from build123d import *

# Parameters (mm, degrees)
F1_DEPTH = 25.4
F3_DEPTH = 25.4
F4_DEPTH = 25.4
F5_R     = 4
F6_DEPTH = 38.1
F7_R     = 7.5
F8_DEPTH = 254


with BuildPart() as f1:
    # F0 (on Top) → F1 (new body)
    with BuildSketch(Plane.XY):
        Polygon((0, 103.923048), (-60, 0), (60, 0), align=None)
    extrude(amount=F1_DEPTH)

    # F2 (on face) → F3 (join)
    with BuildSketch(Plane.XY.offset(25.4)):
        Polygon((12.7, 103.923048), (0, 103.923048), (12.7, 81.926003), align=None)
        Polygon((66.35, 10.998523), (47.3, 21.997045), (60, 0), align=None)
        Polygon((-60, 0), (-47.3, 21.997045), (-66.35, 10.998523), align=None)
        Polygon((-53.65, -10.998523), (-34.6, 0), (-60, 0), align=None)
        Polygon((12.7, 81.926003), (0, 103.923048), (-12.7, 81.926003), align=None)
        Polygon((60, 0), (47.3, 21.997045), (34.6, 0), align=None)
        Polygon((-34.6, 0), (-47.3, 21.997045), (-60, 0), align=None)
        Polygon((60, 0), (34.6, 0), (53.65, -10.998523), align=None)
        Polygon((-12.7, 81.926003), (0, 103.923048), (-12.7, 103.923048), align=None)
    extrude(amount=F3_DEPTH)

    # F2 (on face) → F4 (join)
    with BuildSketch(Plane.XY.offset(25.4)):
        Polygon((12.7, 103.923048), (0, 103.923048), (-12.7, 103.923048), (-12.7, 81.926003), (12.7, 81.926003), align=None)
        Polygon((53.65, -10.998523), (60, 0), (66.35, 10.998523), (47.3, 21.997045), (34.6, 0), align=None)
        Polygon((-66.35, 10.998523), (-60, 0), (-53.65, -10.998523), (-34.6, 0), (-47.3, 21.997045), align=None)
    extrude(amount=-F4_DEPTH)

    # F5 (on face) → F6 (cut)
    with BuildSketch(Plane.XY.offset(50.8)):
        with Locations((0, 92.924526)):
            Circle(F5_R)
        with Locations((-50.475, 5.499261)):
            Circle(F5_R)
        with Locations((50.475, 5.499261)):
            Circle(F5_R)
    extrude(amount=-F6_DEPTH, mode=Mode.SUBTRACT)

    # F7 (on face) → F8 (cut)
    with BuildSketch(Plane.XY.offset(50.8)):
        with Locations((0, 34.641016)):
            Circle(F7_R)
    extrude(amount=-F8_DEPTH, mode=Mode.SUBTRACT)


solid = f1.part
For this review, take the finished solid that the model builds, in its own axes (mm). A direction names the side the tool comes from. Give positions to 0.01 mm unless a question says otherwise; leave off trailing zeros. Loops run counter-clockwise (first coordinate to the right, second up) from the corner with the lowest first, then second, coordinate; pieces in that order, holes last. Notation, with made-up numbers: M 57.25,12.5 L 68.25,12.5 A22 ccw 68.25,20.5 Z; hole C -32.5,82 d9. An arc over 180 degrees is marked long. Put each result on its own line as item: value. Start each with the question number.
(1) Machinability: for faces 5 (the flat face through (-44.3, -5.6, 25.8)), 6 (the flat face through (41.039, 11.153, 37.922)), 7 (the cylindrical face through (46.48, 5.68, 32.02)), 8 (the flat face through (0, 81.926, 38)), which of the approach directions +Z, -Z, +X, -X, +Y, -Y give a long, thin tool a straight path to every point of the face, cutting with its end or side? Answer none if there is none.
(2) Add section D-D, the plane z = 9.5. Write out the cut boundary in (x, y).
(3) Add section A-A, the plane x = 0. Write out the cut boundary in (y, z), then the cut area to 3 significant figures.
(4) For pin 1 (9 mm diameter, centred on x = 0, y = 92.92, fed in from -Z); pin 2 (20.5 mm diameter, centred on x = 0, z = 38, fed in from -Y); pin 3 (12 mm diameter, centred on x = -35, y = 65.5, fed in from +Z); pin 4 (2 mm diameter, centred on x = -25.5, y = 57.5, fed in from +Z), all flat-tipped, find the tip position at first contact; note any pin that passes through.
(5) Add section C-C, the plane y = 40. Write out the cut boundary in (x, z), then the cut area to 3 significant figures.
(6) Wall thickness on L1, parallel to X at y = 5, z = 13.5; L2, parallel to X at y = 8, z = 40.5; L3, parallel to X at y = 87, z = 10: over which ranges is each line inside the solid? List them lowest first.
(7) Add section B-B, the plane z = 40.5. Write out the cut boundary in (x, y) (3 decimals).
(8) The part is to be moulded in two halves that separate along Y. For faces 1 (the flat face through (-47, 2, 50.8)), 2 (the cylindrical face through (1.85, 89.38, 32.02)), 3 (the flat face through (0, 93, 12.7)), 4 (the flat face through (30.242, 51.542, 12.522)), say which applies: +Y half, -Y half, draft (parallel to the pull), parting line (faces both ways), or undercut.
Result:
1. face 5: +Z, -Z, -Y
1. face 6: +Z, +Y
1. face 7: +Z
1. face 8: +Z, +X, -X, -Y
2. outline: M -66.35,11 L -53.65,-11 L -34.6,0 L 34.6,0 L 53.65,-11 L 66.35,11 L 47.3,22 L 12.7,81.93 L 12.7,103.92 L -12.7,103.92 L -12.7,81.93 L -47.3,22 Z; hole C 0,34.64 d15
3. outline: M 0,0 L 27.14,0 L 27.14,25.4 L 0,25.4 Z; M 42.14,0 L 103.92,0 L 103.92,50.8 L 96.92,50.8 L 96.92,12.7 L 88.92,12.7 L 88.92,50.8 L 81.93,50.8 L 81.93,25.4 L 42.14,25.4 Z
3. area: 2,510 mm^2
4. pin 1: stops at z = 0
4. pin 2: stops at y = 81.93
4. pin 3: passes through
4. pin 4: stops at z = 25.4
5. outline: M -36.91,0 L -5.25,0 L -5.25,25.4 L -36.91,25.4 Z; M 5.25,0 L 36.91,0 L 36.91,25.4 L 5.25,25.4 Z
5. area: 1,610 mm^2
6. L1: x = -62.89 to -54.44, -46.51 to 46.51, 54.44 to 62.89
6. L2: x = -64.62 to -53.6, -47.35 to -39.22, 39.22 to 47.35, 53.6 to 64.62
6. L3: x = -12.7 to 12.7
7. outline: M -66.35,10.999 L -53.65,-10.999 L -34.6,0 L -47.3,21.997 Z; M -12.7,81.926 L 12.7,81.926 L 12.7,103.923 L -12.7,103.923 Z; M 34.6,0 L 53.65,-10.999 L 66.35,10.999 L 47.3,21.997 Z; hole C -50.475,5.499 d8; hole C 0,92.925 d8; hole C 50.475,5.499 d8
8. face 1: draft
8. face 2: undercut
8. face 3: undercut
8. face 4: +Y half
